Work out the finished part from the listing and answer in its coordinate system (mm). A direction names the side the tool comes from. Round coordinates to 2 decimals unless told otherwise and drop trailing zeros. Order: outer loops, then holes, each group sorted by start corner. A loop starts at its lowest first (then second) coordinate and runs counter-clockwise, first axis right, second up. Notation, with made-up numbers: (64.5, 82) -> (104.5, 82) arc R33 cw to (104.5, 114) -> close; hole circle Ø4 at (19, 61.25). An arc over 180 degrees is marked (long way). Use one line per item in the form item = value.
```python
from build123d import *

# Parameters (mm, degrees)
SKETCH1_W                     = 60
SKETCH1_H                     = 2
EXTRUDE_THIN1_DEPTH           = 20
SKETCH2_W                     = 1
SKETCH2_H                     = 32
EXTRUDE_THIN2_DEPTH           = 12
SKETCH3_R                     = 1.5
CUT_EXTRUDE1_DEPTH            = 65.373907758
SKETCH4_W                     = 10
SKETCH4_H                     = 2
BOSS_EXTRUDE1_DEPTH           = 2
BOSS_EXTRUDE1_DRAFT           = 2
BOSS_EXTRUDE1_PROFILE_2_DEPTH = 2
BOSS_EXTRUDE1_PROFILE_2_DRAFT = 2
SKETCH6_R                     = 2.5
CUT_EXTRUDE4_DEPTH            = 1
CUT_EXTRUDE4_DRAFT            = 10
CUT_EXTRUDE4_PROFILE_2_DEPTH  = 1
CUT_EXTRUDE4_PROFILE_2_DRAFT  = 10
SKETCH7_R                     = 2.5
CUT_EXTRUDE6_DEPTH            = 1
CUT_EXTRUDE6_DRAFT            = 10
CUT_EXTRUDE7_REACH            = 73.162
SKETCH8_W                     = 4.5
SKETCH8_H                     = 6.050990024
CUT_EXTRUDE8_REACH            = 73.162
SKETCH9_W                     = 4.5
SKETCH9_H                     = 5.78600983
FILLET1_R                     = 0.5


with BuildPart() as part:
    # Sketch1 → Extrude-Thin1 (new, symmetric)
    with BuildSketch(Plane(origin=(0, 0, 0), x_dir=(0, 0, -1), z_dir=(1, 0, 0))):
        with Locations((-30, 1)):
            Rectangle(SKETCH1_W, SKETCH1_H)
    extrude(amount=EXTRUDE_THIN1_DEPTH, both=True)

    # Sketch2 → Extrude-Thin2 (add)
    with BuildSketch(Plane(origin=(0, 2, 0), x_dir=(1, 0, 0), z_dir=(0, 1, 0))):
        with Locations((11.5, -44)):
            Rectangle(SKETCH2_W, SKETCH2_H)
        Polygon((11, -10), (-11, -10), (-11, -60), (-12, -60), (-12, -9), (11, -9), align=None)
    extrude(amount=EXTRUDE_THIN2_DEPTH)

    # Sketch3 → Cut-Extrude1 (cut, through all)
    with BuildSketch(Plane(origin=(0, 2, 0), x_dir=(1, 0, 0), z_dir=(0, 1, 0))):
        with Locations(Location((-16, -5, 0), (0, 0, 270))):
            Circle(SKETCH3_R)
        with Locations(Location((16, -5, 0), (0, 0, 270))):
            Circle(SKETCH3_R)
    extrude(amount=-CUT_EXTRUDE1_DEPTH, mode=Mode.SUBTRACT)


with BuildPart() as boss_extrude1_tool:
    # Sketch4 → Boss-Extrude1 (with draft: the straight prism first)
    with BuildSketch(Plane.XY.offset(60)):
        with Locations((-15, 1)):
            Rectangle(SKETCH4_W, SKETCH4_H)
    extrude(amount=BOSS_EXTRUDE1_DEPTH)
    # Boss-Extrude1: the draft: its side faces are tilted about the plane it starts from
    boss_extrude1_sides = [boss_extrude1_tool.faces().sort_by_distance(p)[0] for p in [
        (-20, 1, 61),
        (-15, 0, 61),
        (-10, 1, 61),
        (-15, 2, 61),
    ]]
    draft(boss_extrude1_sides, Plane.XY.offset(60), BOSS_EXTRUDE1_DRAFT)


with BuildPart() as part_1:
    add(part.part)

    # Boss-Extrude1: add boss_extrude1_tool
    add(boss_extrude1_tool.part)


with BuildPart() as boss_extrude1_profile_2_tool:
    # Sketch4 → Boss-Extrude1 profile 2 (with draft: the straight prism first)
    with BuildSketch(Plane.XY.offset(60)):
        with Locations((15, 1)):
            Rectangle(SKETCH4_W, SKETCH4_H)
    extrude(amount=BOSS_EXTRUDE1_PROFILE_2_DEPTH)
    # Boss-Extrude1 profile 2: the draft: its side faces are tilted about the plane it starts from
    boss_extrude1_profile_2_sides = [boss_extrude1_profile_2_tool.faces().sort_by_distance(p)[0] for p in [
        (10, 1, 61),
        (15, 0, 61),
        (20, 1, 61),
        (15, 2, 61),
    ]]
    draft(boss_extrude1_profile_2_sides, Plane.XY.offset(60), BOSS_EXTRUDE1_PROFILE_2_DRAFT)


with BuildPart() as part_2:
    add(part_1.part)

    # Boss-Extrude1 profile 2: add boss_extrude1_profile_2_tool
    add(boss_extrude1_profile_2_tool.part)


with BuildPart() as cut_extrude4_tool:
    # Sketch6 → Cut-Extrude4 (with draft: the straight prism first)
    with BuildSketch(Plane(origin=(12, 0, 0), x_dir=(0, 0, -1), z_dir=(1, 0, 0))):
        with Locations((-55, 9.5)):
            Circle(SKETCH6_R)
    extrude(amount=-CUT_EXTRUDE4_DEPTH)
    # Cut-Extrude4: the draft: its side faces are tilted about the plane it starts from
    cut_extrude4_sides = [cut_extrude4_tool.faces().sort_by_distance(p)[0] for p in [
        (11.5, 9.5, 57.5),
    ]]
    draft(cut_extrude4_sides, Plane(origin=(12, 0, 0), x_dir=(0, 0, -1), z_dir=(1, 0, 0)), CUT_EXTRUDE4_DRAFT)


with BuildPart() as part_3:
    add(part_2.part)

    # Cut-Extrude4: cut by cut_extrude4_tool
    add(cut_extrude4_tool.part, mode=Mode.SUBTRACT)


with BuildPart() as cut_extrude4_profile_2_tool:
    # Sketch6 → Cut-Extrude4 profile 2 (with draft: the straight prism first)
    with BuildSketch(Plane(origin=(12, 0, 0), x_dir=(0, 0, -1), z_dir=(1, 0, 0))):
        with Locations((-43.5, 9.5)):
            Circle(SKETCH6_R)
    extrude(amount=-CUT_EXTRUDE4_PROFILE_2_DEPTH)
    # Cut-Extrude4 profile 2: the draft: its side faces are tilted about the plane it starts from
    cut_extrude4_profile_2_sides = [cut_extrude4_profile_2_tool.faces().sort_by_distance(p)[0] for p in [
        (11.5, 9.5, 46),
    ]]
    draft(cut_extrude4_profile_2_sides, Plane(origin=(12, 0, 0), x_dir=(0, 0, -1), z_dir=(1, 0, 0)), CUT_EXTRUDE4_PROFILE_2_DRAFT)


with BuildPart() as part_4:
    add(part_3.part)

    # Cut-Extrude4 profile 2: cut by cut_extrude4_profile_2_tool
    add(cut_extrude4_profile_2_tool.part, mode=Mode.SUBTRACT)


with BuildPart() as cut_extrude6_tool:
    # Sketch7 → Cut-Extrude6 (with draft: the straight prism first)
    with BuildSketch(Plane.ZY.offset(12)):
        with Locations((53.5, 9.5)):
            Circle(SKETCH7_R)
    extrude(amount=-CUT_EXTRUDE6_DEPTH)
    # Cut-Extrude6: the draft: its side faces are tilted about the plane it starts from
    cut_extrude6_sides = [cut_extrude6_tool.faces().sort_by_distance(p)[0] for p in [
        (-11.5, 9.5, 51),
    ]]
    draft(cut_extrude6_sides, Plane.ZY.offset(12), CUT_EXTRUDE6_DRAFT)


with BuildPart() as part_5:
    add(part_4.part)

    # Cut-Extrude6: cut by cut_extrude6_tool
    add(cut_extrude6_tool.part, mode=Mode.SUBTRACT)

    # Sketch8 → Cut-Extrude7 (cut, up to next)
    with BuildSketch(Plane(origin=(12, 0, 0), x_dir=(0, 0, -1), z_dir=(1, 0, 0)), mode=Mode.PRIVATE) as cut_extrude7_sk1:
        with Locations((-55, 12.491774439)):
            Rectangle(SKETCH8_W, SKETCH8_H)
    cut_extrude7_tool1 = extrude(cut_extrude7_sk1.sketch, amount=-CUT_EXTRUDE7_REACH, mode=Mode.PRIVATE) & part_5.part
    # Sketch8 → Cut-Extrude7 (cut, up to next)
    with BuildSketch(Plane(origin=(12, 0, 0), x_dir=(0, 0, -1), z_dir=(1, 0, 0)), mode=Mode.PRIVATE) as cut_extrude7_sk2:
        with Locations((-43.5, 12.460513527)):
            Rectangle(SKETCH8_W, SKETCH8_H)
    cut_extrude7_tool2 = extrude(cut_extrude7_sk2.sketch, amount=-CUT_EXTRUDE7_REACH, mode=Mode.PRIVATE) & part_5.part
    add(cut_extrude7_tool1.solids().sort_by_distance((12, 12.491774, 55))[0], mode=Mode.SUBTRACT)
    add(cut_extrude7_tool2.solids().sort_by_distance((12, 12.460514, 43.5))[0], mode=Mode.SUBTRACT)

    # Sketch9 → Cut-Extrude8 (cut, up to next)
    with BuildSketch(Plane.ZY.offset(12), mode=Mode.PRIVATE) as cut_extrude8_sk1:
        with Locations((53.5, 13.082945191)):
            Rectangle(SKETCH9_W, SKETCH9_H)
    cut_extrude8_tool1 = extrude(cut_extrude8_sk1.sketch, amount=-CUT_EXTRUDE8_REACH, mode=Mode.PRIVATE) & part_5.part
    add(cut_extrude8_tool1.solids().sort_by_distance((-12, 13.082945, 53.5))[0], mode=Mode.SUBTRACT)

    # Fillet1
    fillet1_edges = [part_5.edges().sort_by_distance(p)[0] for p in [
        (11.5, 14, 52.75),
        (11.5, 14, 57.25),
        (11.5, 14, 41.25),
        (11.5, 14, 45.75),
        (-11.5, 14, 55.75),
        (-11.5, 14, 51.25),
    ]]
    fillet(fillet1_edges, radius=FILLET1_R)


solid = part_5.part
```
Item 1: Consider line 1 along X through (y, z) = (1.3, 5); line 2 along X through (y, z) = (8.25, 36); line 3 along Y through (x, z) = (-2, 6). Determine where each line is inside the solid, lowest interval first.
Findings:
line_1 = -20 to -17.5, -14.5 to 14.5, 17.5 to 20
line_2 = -12 to -11, 11 to 12
line_3 = 0 to 2
Item 2: Flat-ended cylindrical pins translate along their axes: P1, Ø5, axis at x = -10.5, y = 9.5, coming from the -Z side; P2, Ø8, axis at x = 5, y = 10, coming from the +Z side; P3, Ø2.5, axis at x = -16, z = 5, coming from the +Y side; P4, Ø0.8, axis at x = -11.5, y = 12.5, coming from the +Z side. Find the tip coordinate at first contact, or state that the pin passes through.
Findings:
P1 = 9
P2 = 10
P3 = through
P4 = 60
Item 3: The part is cut by section A-A, the plane x = -16. Give the vertices of the cut face in (y, z), and give its area (3 significant figures).
Findings:
outline = (0, 0) -> (2, 0) -> (2, 3.5) -> (0, 3.5) -> close; (0, 6.5) -> (2, 6.5) -> (2, 60) -> (1.93, 62) -> (0.07, 62) -> (0, 60) -> close
area = 118 mm^2
Item 4: The part is cut by section C-C, the plane z = 12.5. Give the vertices of the cut face in (x, y), and give its area (3 significant figures).
Findings:
outline = (-20, 0) -> (20, 0) -> (20, 2) -> (-11, 2) -> (-11, 14) -> (-12, 14) -> (-12, 2) -> (-20, 2) -> close
area = 92.0 mm^2
Item 5: The part is cut by section B-B, the plane y = 9.5. Give the vertices of the cut face in (x, z), and give its area (3 significant figures).
Findings:
outline = (-12, 9) -> (11, 9) -> (11, 10) -> (-11, 10) -> (-11, 50.82) -> (-12, 51) -> close; (-12, 56) -> (-11, 56.18) -> (-11, 60) -> (-12, 60) -> close; (11, 28) -> (12, 28) -> (12, 41) -> (11, 40.82) -> close; (11, 46.18) -> (12, 46) -> (12, 52.5) -> (11, 52.32) -> close; (11, 57.68) -> (12, 57.5) -> (12, 60) -> (11, 60) -> close
area = 89.5 mm^2
Item 6: Determine the mould class of faces 1 (the flat face through (-1, 8, 9)), 2 (the flat face through (-20, 1, 30)), 3 (the conical face through (11.729, 6.953, 55.076)), 4 (the cylindrical face through (-15.55, 1.01, 6.43)) for opening direction X: released by +X, released by -X, zero draft, split by the parting line, or undercut.
Findings:
face_1 = zero draft
face_2 = released by -X
face_3 = undercut
face_4 = undercut
Item 7: For faces 5 (the flat face through (0, 8, 10)), 6 (the flat face through (12, 6.6, 44.2)), 7 (the flat face through (-12, 8, 35)), determine the directions among +Z, -Z, +X, -X, +Y, -Y from which every point of the face is accessible in a straight line to the end or side of a thin tool.
Findings:
face_5 = +Z, +X, +Y
face_6 = +Z, -Z, +X, +Y
face_7 = +Z, -Z, -X, +Y
Item 8: The part is cut by section D-D, the plane y = 3. Give the vertices of the cut face in (x, z).
Findings:
outline = (-12, 9) -> (11, 9) -> (11, 10) -> (-11, 10) -> (-11, 60) -> (-12, 60) -> close; (11, 28) -> (12, 28) -> (12, 60) -> (11, 60) -> close
